Could you check a few things on this model? Use its own coordinates, in mm. A direction names the side the tool comes from. Give positions to 0.01 mm unless a question says otherwise; leave off trailing zeros. Loops run counter-clockwise (first coordinate to the right, second up) from the corner with the lowest first, then second, coordinate; pieces in that order, holes last. Notation, with made-up numbers: (54, -8.5) -> (70, -8.5) arc R21 ccw to (70, 20.5) -> close; hole circle Ø4 at (34, 39). An arc over 180 degrees is marked (long way). Put each result on its own line as item: value.
```python
from build123d import *

# Parameters (mm, degrees)
BOSS_EXTRUDE1_DEPTH = 20
FILLET1_R           = 10
SKETCH2_R           = 3.175
CUT_EXTRUDE1_DEPTH  = 21
SKETCH3_R           = 3.175
CUT_EXTRUDE2_DEPTH  = 4


with BuildPart() as part:
    # Sketch1 → Boss-Extrude1 (new body)
    with BuildSketch(Plane(origin=(0, 0, 0), x_dir=(1, 0, 0), z_dir=(0, 1, 0))):
        Polygon((-18.5, -1.5), (-1.5, -1.5), (-1.5, -18.5), (1.5, -18.5), (1.5, 1.5), (-18.5, 1.5), align=None)
    extrude(amount=BOSS_EXTRUDE1_DEPTH)

    # Fillet1
    fillet1_edges = [part.edges().sort_by_distance(p)[0] for p in [
        (0, 20, 18.5),
        (-18.5, 20, 0),
    ]]
    fillet(fillet1_edges, radius=FILLET1_R)

    # Sketch2 → Cut-Extrude1 (cut, through all)
    with BuildSketch(Plane(origin=(1.5, 0, 0), x_dir=(0, 0, -1), z_dir=(1, 0, 0))):
        with Locations((-11.5, 13)):
            Circle(SKETCH2_R)
    extrude(amount=-CUT_EXTRUDE1_DEPTH, mode=Mode.SUBTRACT)

    # Sketch3 → Cut-Extrude2 (cut, through all)
    with BuildSketch(Plane.XY.offset(1.5)):
        with Locations((-11.5, 13)):
            Circle(SKETCH3_R)
    extrude(amount=-CUT_EXTRUDE2_DEPTH, mode=Mode.SUBTRACT)


solid = part.part
```
1. If we section it at D-D (z = 0.5): List the corners of the cut face in (x, y) for me (3 decimals), then the cut area to 3 significant figures.
Recorded:
outline: (-18.5, 0) -> (1.5, 0) -> (1.5, 20) -> (-8.5, 20) arc R10 ccw to (-18.5, 10) -> close; hole circle Ø6.35 at (-11.5, 13)
area: 347 mm^2
2. I need wall thicknesses on line 1 (Z direction, x = -1.75, y = 12); line 2 (Y direction, x = -11.5, z = 0.05) (3 decimals); line 3 (Y direction, x = -0.25, z = 10). Which ranges of each line are inside material? Lowest first, please.
Recorded:
line 1: z = -1.5 to 1.5
line 2: y = 0 to 9.825, 16.175 to 19.539
line 3: y = 0 to 10.2, 15.8 to 19.89
3. For faces 1 (the face through (-18.5, 5, 0)), 2 (the face through (-10, 10, 1.5)), which set-ups out of +Z, -Z, +X, -X, +Y, -Y let a thin tool reach every point of the face, with its end or its side?
Recorded:
face 1: +Z, -Z, -X, +Y, -Y
face 2: +Z, -X, +Y, -Y
4. If we section it at C-C (x = -11.5): List the corners of the cut face in (y, z) for me (3 decimals), then the cut area to 3 significant figures.
Recorded:
outline: (0, -1.5) -> (9.825, -1.5) -> (9.825, 1.5) -> (0, 1.5) -> close; (16.175, -1.5) -> (19.539, -1.5) -> (19.539, 1.5) -> (16.175, 1.5) -> close
area: 39.6 mm^2
5. Thinking about a two-plate mould opening in X: for faces 3 (the face through (-1, 20, 2)), 4 (the face through (-15.65, 16.99, 0.02)), 5 (the face through (-11.91, 16.15, 0.02)), which applies, pulls with the +X half, pulls with the -X half, needs draft (parallel to the pull), parting line crosses it, or undercut?
Recorded:
face 3: needs draft
face 4: pulls with the -X half
face 5: undercut
6. If we section it at A-A (z = 11.5): List the corners of the cut face in (x, y) for me (3 decimals).
Recorded:
outline: (-1.5, 0) -> (1.5, 0) -> (1.5, 9.825) -> (-1.5, 9.825) -> close; (-1.5, 16.175) -> (1.5, 16.175) -> (1.5, 19.539) -> (-1.5, 19.539) -> close
7. If we section it at B-B (y = 11.5): List the corners of the cut face in (x, z) for me, then the cut area to 3 significant figures.
Recorded:
outline: (-18.39, -1.5) -> (-14.3, -1.5) -> (-14.3, 1.5) -> (-18.39, 1.5) -> close; (-8.7, -1.5) -> (1.5, -1.5) -> (1.5, 8.7) -> (-1.5, 8.7) -> (-1.5, 1.5) -> (-8.7, 1.5) -> close; (-1.5, 14.3) -> (1.5, 14.3) -> (1.5, 18.39) -> (-1.5, 18.39) -> close
area: 76.7 mm^2
8. I'm going to push flat-ended pins straight in: pin 1 (5 mm diameter, centred on x = -11.5, y = 13, fed in from -Z); pin 2 (10 mm diameter, centred on y = 13, z = 11.5, fed in from -X); pin 3 (10 mm diameter, centred on x = -15, y = 13, fed in from +Z); pin 4 (8 mm diameter, centred on x = -3.5, y = 14.5, fed in from +Z). Where does each tip first touch, or does it pass through?
Recorded:
pin 1: passes through
pin 2: stops at x = -1.5
pin 3: stops at z = 1.5
pin 4: stops at z = 18.45
